Work out the finished part from the listing and answer in its coordinate system (mm). A direction names the side the tool comes from. Round coordinates to 2 decimals unless told otherwise and drop trailing zeros. Loops run counter-clockwise (first coordinate to the right, second up) from the corner with the lowest first, then second, coordinate; pieces in that order, holes last. Notation, with made-up numbers: M -24.5,-4.5 L 17.5,-4.5 A18 ccw 17.5,27.5 Z; hole C -31.5,24 d1. An arc over 180 degrees is marked long. One line per item, written item: value.
```python
from build123d import *

# Parameters (mm, degrees)
SKETCH_1_W          = 110
SKETCH_1_H          = 52
EXTRUDE_1_DEPTH     = 25
SKETCH_2_R          = 1.25
CUT_EXTRUDE_1_DEPTH = 6
SKETCH_3_W          = 4
SKETCH_3_H          = 10
CUT_EXTRUDE_2_DEPTH = 6
SKETCH_4_W          = 4
SKETCH_4_H          = 10
CUT_EXTRUDE_3_DEPTH = 6
SKETCH_5_W          = 17
SKETCH_5_H          = 8
CUT_EXTRUDE_4_DEPTH = 2
FILLET_1_R          = 3


with BuildPart() as part:
    # Эскиз1 → Бобышка-Вытянуть1 (new body)
    with BuildSketch(Plane.XY):
        with Locations((55, 26)):
            Rectangle(SKETCH_1_W, SKETCH_1_H)
    extrude(amount=EXTRUDE_1_DEPTH)

    # Эскиз2 → Вырез-Вытянуть1 (cut)
    with BuildSketch(Plane(origin=(110, 0, 0), x_dir=(0, 0, -1), z_dir=(1, 0, 0))):
        with BuildLine():
            Line((-9.5, 31), (-9.5, 21))
            ThreePointArc((-9.5, 21), (-12.5, 18), (-15.5, 21))
            Line((-15.5, 21), (-15.5, 31))
            ThreePointArc((-15.5, 31), (-12.5, 34), (-9.5, 31))
        make_face()
        with Locations(Location((-12.5, 29, 0), (0, 0, 90))):
            Circle(SKETCH_2_R, mode=Mode.SUBTRACT)
        with Locations(Location((-12.5, 23, 0), (0, 0, 90))):
            Circle(SKETCH_2_R, mode=Mode.SUBTRACT)
    extrude(amount=-CUT_EXTRUDE_1_DEPTH, mode=Mode.SUBTRACT)

    # Эскиз3 → Вырез-Вытянуть2 (cut)
    with BuildSketch(Plane.ZY):
        with Locations((12.5, 9)):
            Rectangle(SKETCH_3_W, SKETCH_3_H)
    extrude(amount=-CUT_EXTRUDE_2_DEPTH, mode=Mode.SUBTRACT)

    # Эскиз4 → Вырез-Вытянуть3 (cut)
    with BuildSketch(Plane.ZY):
        with Locations((12.5, 43)):
            Rectangle(SKETCH_4_W, SKETCH_4_H)
    extrude(amount=-CUT_EXTRUDE_3_DEPTH, mode=Mode.SUBTRACT)

    # Эскиз5 → Вырез-Вытянуть4 (cut)
    with BuildSketch(Plane(origin=(0, 0, 0), x_dir=(-1, 0, 0), z_dir=(0, 0, -1))):
        with Locations((-23.5, 9)):
            Rectangle(SKETCH_5_W, SKETCH_5_H)
    extrude(amount=-CUT_EXTRUDE_4_DEPTH, mode=Mode.SUBTRACT)

    # Скругление1
    fillet_1_edges = [part.edges().sort_by_distance(p)[0] for p in [
        (110, 26, 25),
        (55, 52, 25),
        (0, 26, 25),
        (55, 52, 0),
        (110, 26, 0),
        (55, 0, 0),
        (0, 26, 0),
        (55, 0, 25),
        (0, 52, 12.5),
        (110, 52, 12.5),
        (110, 0, 12.5),
        (0, 0, 12.5),
    ]]
    fillet(fillet_1_edges, radius=FILLET_1_R)


solid = part.part
```
1) The mould has two halves that part along Y. Classify faces 6 (the face through (3, 43, 10.5)), 7 (the face through (55.73, 0.86, 24.1)), 8 (the face through (0, 26, 12)): +Y half, -Y half, draft (parallel to the pull), parting line (faces both ways), or undercut.
Check values:
face 6: undercut
face 7: -Y half
face 8: draft
2) For faces 1 (the face through (110, 29, 12)), 2 (the face through (32, 9, 1)), 3 (the face through (3, 9, 10.5)), 4 (the face through (0.86, 26.32, 24.1)), 5 (the face through (107, 18, 12.4)), determine the directions among +Z, -Z, +X, -X, +Y, -Y from which every point of the face is accessible in a straight line to the end or side of a thin tool.
Check values:
face 1: +Z, -Z, +X, +Y, -Y
face 2: -Z
face 3: -X
face 4: +Z, -X, +Y, -Y
face 5: +X
3) Each of these flat-tipped pins is pushed along its axis until it touches: pin 1 (1 mm diameter, centred on y = 10.5, z = 1.5, fed in from -X); pin 2 (1 mm diameter, centred on y = 7, z = 0.5, fed in from +X); pin 3 (1.6 mm diameter, centred on x = 22.5, z = 0.5, fed in from -Y). Where does it stop, or does it pass through?
Check values:
pin 1: x = 0.17
pin 2: x = 109.24
pin 3: y = 0.53
4) Find the intervals of material crossed by probe 1 along X at (y, z) = (6, 11.25); probe 2 along Y at (x, z) = (25.5, 23); probe 3 along Y at (x, z) = (8.5, 1.5), in increasing order. Write a range as from..to.
Check values:
probe 1: 6..110
probe 2: 0.17..51.83
probe 3: 0.4..51.6
5) Find section B-B (z = 12.5). Give the vertices of the cut face in (x, y), then the cut area to 3 significant figures.
Check values:
outline: M 0,3 A3 ccw 3,0 L 107,0 A3 ccw 110,3 L 110,18 L 104,18 L 104,21.75 L 110,21.75 L 110,24.25 L 104,24.25 L 104,27.75 L 110,27.75 L 110,30.25 L 104,30.25 L 104,34 L 110,34 L 110,49 A3 ccw 107,52 L 3,52 A3 ccw 0,49 L 0,48 L 6,48 L 6,38 L 0,38 L 0,14 L 6,14 L 6,4 L 0,4 Z
area: 5,530 mm2
6) Find section C-C (x = 25). Give the vertices of the cut face in (y, z), then the cut area to 3 significant figures.
Check values:
outline: M 0,3 A3 ccw 3,0 L 5,0 L 5,2 L 13,2 L 13,0 L 49,0 A3 ccw 52,3 L 52,22 A3 ccw 49,25 L 3,25 A3 ccw 0,22 Z
area: 1,280 mm2
7) Find section A-A (y = 11). Give the vertices of the cut face in (x, z), then the cut area to 3 significant figures.
Check values:
outline: M 0,3 A3 ccw 3,0 L 15,0 L 15,2 L 32,2 L 32,0 L 107,0 A3 ccw 110,3 L 110,22 A3 ccw 107,25 L 3,25 A3 ccw 0,22 L 0,14.5 L 6,14.5 L 6,10.5 L 0,10.5 Z
area: 2,680 mm2
8) Find section D-D (z = 23.25). Give the vertices of the cut face in (x, y), then the cut area to 3 significant figures.
Check values:
outline: M 0.27,3 A2.73 ccw 3,0.27 L 107,0.27 A2.73 ccw 109.73,3 L 109.73,49 A2.73 ccw 107,51.73 L 3,51.73 A2.73 ccw 0.27,49 Z
area: 5,630 mm2
